from build123d import *

# Parameters (mm, degrees)
F1_DEPTH  = 10
F0_R      = 1.55
F2_DEPTH  = 10
F4_DEPTH  = 50
F6_DEPTH  = 4
F7_R      = 1.5
F8_DEPTH  = 5
F9_R      = 1.5
F10_DEPTH = 25
F11_R     = 1.5
F12_DEPTH = 25


# Not quite as in the source:
# - ends of sketch curves that miss each other by under 0.0002 mm in the source are joined


with BuildPart() as f1:
    # F0 (on Front) → F1 (new body, symmetric)
    with BuildSketch(Plane.XZ):
        with BuildLine():
            ThreePointArc((-22.75, 0), (-1.4668388401, 22.702662483), (22.560846929, 2.9275733717))
            Line((22.560846929, 2.9275733717), (25.5830376256, 2.9275733717))
            Line((25.5830376256, 2.9275733717), (47.75, 2.9275733717))
            Line((47.75, 2.9275733717), (47.75, 8.9275733717))
            Line((47.75, 8.9275733717), (41.0830374761, 8.9275733717))
            ThreePointArc((41.0830374761, 8.9275733717), (39.1491782862, 9.316696163), (37.5163225707, 10.4234979182))
            Line((37.5163225707, 10.4234979182), (7.964999938, 40.503085047))
            Line((7.964999938, 40.503085047), (2.164999938, 40.503085047))
            Line((2.164999938, 40.503085047), (2.164999938, 36.703085047))
            Line((2.164999938, 36.703085047), (4.664999938, 36.703085047))
            Line((4.664999938, 36.703085047), (4.664999938, 37.703085047))
            Line((4.664999938, 37.703085047), (6.264999938, 37.703085047))
            Line((6.264999938, 37.703085047), (6.264999938, 31.703085047))
            Line((6.264999938, 31.703085047), (-1.235000062, 31.703085047))
            Line((-1.235000062, 31.703085047), (-8.735000062, 31.7030854494))
            Line((-8.735000062, 31.7030854494), (-8.735000062, 37.7030854494))
            Line((-8.735000062, 37.7030854494), (-7.135000062, 37.7030854494))
            Line((-7.135000062, 37.7030854494), (-7.135000062, 36.7030854494))
            Line((-7.135000062, 36.7030854494), (-4.635000062, 36.7030854494))
            Line((-4.635000062, 36.7030854494), (-4.635000062, 40.5030854494))
            Line((-4.635000062, 40.5030854494), (-9.0264711097, 40.5030854494))
            ThreePointArc((-9.0264711097, 40.5030854494), (-10.3822316524, 40.3157680019), (-11.6364091533, 39.7678507898))
            Line((-11.6364091533, 39.7678507898), (-55.7125058122, 12.7942960211))
            ThreePointArc((-55.7125058122, 12.7942960211), (-40.5494526959, 13.0852438258), (-32.8826916814, 0))
            Line((-32.8826916814, 0), (-25.75, 0))
            Line((-25.75, 0), (-22.75, 0))
        make_face()
    extrude(amount=F1_DEPTH, both=True)

    # F0 (on Front) → F2 (join)
    with BuildSketch(Plane.XZ):
        with BuildLine():
            ThreePointArc((-55.7125058122, 12.7942960211), (-55.2159306669, -13.0852438258), (-32.8826916814, 0))
            ThreePointArc((-32.8826916814, 0), (-40.5494526959, 13.0852438258), (-55.7125058122, 12.7942960211))
        make_face()
        with Locations((-47.8826916814, 0)):
            Circle(F0_R, mode=Mode.SUBTRACT)
    extrude(amount=F2_DEPTH)

    # F3 (on face) → F4 (cut)
    with BuildSketch(Plane(origin=(0, 0, 2.9275733717), x_dir=(1, 0, 0), z_dir=(0, 0, -1))):
        Polygon((42.583, -2.5980762114), (44.083, 0), (42.583, 2.5980762114), (39.583, 2.5980762114), (38.083, 0), (39.583, -2.5980762114), align=None)
    extrude(amount=-F4_DEPTH, mode=Mode.SUBTRACT)

    # F5 (on face) → F6 (join)
    with BuildSketch(Plane(origin=(0, 0, 2.9275733717), x_dir=(1, 0, 0), z_dir=(0, 0, -1))):
        Polygon((42.583, 2.5980762114), (39.583, 2.5980762114), (38.083, 0), (39.583, -2.5980762114), (42.583, -2.5980762114), (44.083, 0), align=None)
    extrude(amount=-F6_DEPTH)

    # F7 (on face) → F8 (cut)
    with BuildSketch(Plane.XY.offset(6.9275733717)):
        with Locations((41.083, 0)):
            Circle(F7_R)
    extrude(amount=-F8_DEPTH, mode=Mode.SUBTRACT)

    # F9 (on face) → F10 (cut)
    with BuildSketch(Plane(origin=(0, 0, 2.9275733717), x_dir=(1, 0, 0), z_dir=(0, 0, -1))):
        Polygon((-4.235000062, 10), (-4.235000062, -10), (-1.235000062, -10), (1.764999938, -10), (1.764999938, 10), align=None)
        with Locations((-1.235000062, 0)):
            Circle(F9_R, mode=Mode.SUBTRACT)
    extrude(amount=-F10_DEPTH, mode=Mode.SUBTRACT)

    # F11 (on face) → F12 (cut)
    with BuildSketch(Plane.XY.offset(31.703085047)):
        with Locations((-1.235000062, 0)):
            Circle(F11_R)
    extrude(amount=-F12_DEPTH, mode=Mode.SUBTRACT)


solid = f1.part
Model file for the job. Use its own axes, mm. A direction names the side the tool comes from. Coordinates: 2 decimals unless noted, no trailing zeros. Write each loop counter-clockwise with the first axis right and the second up, starting at its lowest first coordinate (ties: lowest second). Pieces come first, ordered by that corner, then holes. Notation, with made-up numbers: (51.5, 72.25) - (75.5, 72.25) arc R32 cw to (75.5, 105.25) - close; hole circle Ø4 at (-31, -14). An arc over 180 degrees is marked (long way). Write each question's results on one line, items separated by ' | '. Start each with the question number.
1) Probe line 1 along X through (y, z) = (5, 37.5) (3 decimals); line 2 along X through (y, z) = (0, 30.3) (3 decimals); line 3 along X through (y, z) = (0.5, 37) (3 decimals). List the from-to ranges inside material, lowest first. Write a range as from..to.
2) Mould opens along Y. For faces 6 (the face through (-21, -10, 13)), 7 (the face through (-46.404, -4.93, 0.466)), 8 (the face through (38.82, 1.28, 8.07)) say: pulls with the +Y half, pulls with the -Y half, needs draft (parallel to the pull), parting line crosses it, or undercut.
3) Cut at B-B (z = 21). Write the cut outline in (x, y), then the cut area to 3 significant figures.
4) Flat gauge pins, fed straight in: P1, Ø8, axis at x = -31.5, y = -6, coming from the +Z side; P2, Ø1.5, axis at x = -11, y = 6.5, coming from the +Z side; P3, Ø2, axis at x = -3.5, y = -1, coming from the +Z side. Where does each tip first touch, or does it go through?
5) 3-axis set-ups, long thin cutter, end or side, ignore diameter. For faces 1 (the face through (2.165, 0, 39)), 2 (the face through (42.4, -1.2, 6.928)), 3 (the face through (-17.66, -0.14, 14.34)), 4 (the face through (-40.74, 4.93, 13.19)), 5 (the face through (-6, 0, 36.703)): which of +Z, -Z, +X, -X, +Y, -Y reach the whole face in a straight line?
6) Cut at C-C (z = -5). Write the cut outline in (x, y).
Returned:
1) line 1: -15.342..-8.735, -7.135..-4.635, 2.165..4.665, 6.265..10.915 | line 2: -27.107..-2.735, 0.265..17.989 | line 3: -16.159..-8.735, -7.135..-4.635, 2.165..4.665, 6.265..11.407
2) face 6: pulls with the -Y half | face 7: needs draft | face 8: undercut
3) outline: (-42.3, -10) - (-8.75, -10) - (-8.75, 10) - (-42.3, 10) - close; (8.75, -10) - (27.13, -10) - (27.13, 10) - (8.75, 10) - close | area: 1,040 mm^2
4) P1: z = 30.06 | P2: z = 40.35 | P3: z = 31.7
5) face 1: +Z, +Y, -Y | face 2: +Z | face 3: -Z, +Y, -Y | face 4: -Z, +Y | face 5: +Y, -Y
6) outline: (-62.02, -10) - (-33.74, -10) - (-33.74, 0) - (-62.02, 0) - close
